```python
from build123d import *

# Parameters (mm, degrees)
F0_R     = 28.575
F1_DEPTH = 40.2336
F2_R     = 3.302
F4_DEPTH = 40.2336


with BuildPart() as f1:
    # F0 (on Top) → F1 (new body)
    with BuildSketch(Plane.XY):
        Circle(F0_R)
    extrude(amount=F1_DEPTH)

    # F2
    f2_edges = [f1.edges().sort_by_distance(p)[0] for p in [
        (-28.575, 0, 40.2336),
    ]]
    fillet(f2_edges, radius=F2_R)

    # F3 (on face) → F4 (cut, through all)
    with BuildSketch(Plane.XY.offset(40.2336)):
        with BuildLine():
            Line((18.5293, 4.826), (13.447765, 4.826))
            ThreePointArc((13.447765, 4.826), (-14.2875, 0), (13.447765, -4.826))
            Line((13.447765, -4.826), (18.5293, -4.826))
            Line((18.5293, -4.826), (18.5293, 4.826))
        make_face()
    extrude(amount=-F4_DEPTH, mode=Mode.SUBTRACT)


solid = f1.part
```
Work out the finished part from the listing and answer in its coordinate system (mm). A direction names the side the tool comes from. Round coordinates to 2 decimals unless told otherwise and drop trailing zeros. Write each loop counter-clockwise with the first axis right and the second up, starting at its lowest first coordinate (ties: lowest second). Pieces come first, ordered by that corner, then holes.
1) A cutting plane is placed at D-D on z = 38. Determine the outline of the cut face in (x, y) (1 decimal).
2) A cutting plane is placed at A-A on x = 0. Determine the outline of the cut face in (y, z) (1 decimal).
3) Which of the six approach directions +Z, -Z, +X, -X, +Y, -Y give full straight-line access (tool end or side, diameter ignored) to faces 1 (the face through (11, -11, 40.234)), 2 (the face through (16, -4.826, 20))?
4) A cutting plane is placed at B-B on y = 0. Determine the outline of the cut face in (x, z) (1 decimal), and give its area (3 significant figures).
5) Consider probe 1 along Y at (x, z) = (0, 18) (1 decimal); probe 2 along Y at (x, z) = (10.5, 6.5); probe 3 along X at (y, z) = (-8, 27.5). Determine where each line is inside the solid, lowest interval first.
6) Flat-ended cylindrical pins translate along their axes: P1, Ø12, axis at x = -15.5, z = 19, coming from the -Y side; P2, Ø8, axis at y = 8, z = 6.5, coming from the -X side; P3, Ø4, axis at x = 17, z = 16, coming from the -Y side. Find the tip coordinate at first contact, or state that the pin passes through.
7) Determine the mould class of faces 3 (the face through (18.529, 0, 20)), 4 (the face through (-13, 7, 0)), 5 (the face through (-28.547, 1.256, 18.207)) for opening direction X: pulls with the +X half, pulls with the -X half, needs draft (parallel to the pull), parting line crosses it, or undercut.
Entries:
1. outline: circle Ø56.8 at (0, 0); hole (13.4, -4.8) - (18.5, -4.8) - (18.5, 4.8) - (13.4, 4.8) arc R14.3 ccw (long way) to start
2. outline: (-28.6, 0) - (-14.3, 0) - (-14.3, 40.2) - (-25.3, 40.2) arc R3.3 ccw to (-28.6, 36.9) - close; (14.3, 0) - (28.6, 0) - (28.6, 36.9) arc R3.3 ccw to (25.3, 40.2) - (14.3, 40.2) - close
3. face 1: +Z, +X, -X, +Y, -Y
3. face 2: +Z, -Z
4. outline: (-28.6, 0) - (-14.3, 0) - (-14.3, 40.2) - (-25.3, 40.2) arc R3.3 ccw to (-28.6, 36.9) - close; (18.5, 0) - (28.6, 0) - (28.6, 36.9) arc R3.3 ccw to (25.3, 40.2) - (18.5, 40.2) - close
4. area: 974 mm2
5. probe 1: y = -28.6 to -14.3, 14.3 to 28.6
5. probe 2: y = -26.58 to -9.69, 9.69 to 26.58
5. probe 3: x = -27.43 to -11.84, 11.84 to 27.43
6. P1: stops at y = -26.95
6. P2: stops at x = -28.29
6. P3: stops at y = -24.32
7. face 3: undercut
7. face 4: needs draft
7. face 5: parting line crosses it
